Verification items for the finished model (mm, model axes). Face numbers are marked on the shaded views. A direction names the side the tool comes from. Give positions to 0.01 mm unless a question says otherwise; leave off trailing zeros. Loops run counter-clockwise (first coordinate to the right, second up) from the corner with the lowest first, then second, coordinate; pieces in that order, holes last. Notation, with made-up numbers: (80, 48) -> (133, 48) arc R31 cw to (133, 77) -> close; hole circle Ø4 at (79, 35.25). An arc over 180 degrees is marked (long way). Answer in a Markdown table with one row per item. Add a question column.
Q1. Gauge pin test, flat ends, axial feed: P1, Ø7.5, axis at x = 15.5, y = -41.5, coming from the -Z side; P2, Ø1.8, axis at x = 17, y = -42.5, coming from the +Z side; P3, Ø2, axis at x = -16.5, y = -1, coming from the -Z side; P4, Ø5, axis at y = -26.5, z = 3.5, coming from the +X side. Record the tip position at first contact, or that the pin passes through.
Q2. Material ranges on probe 1 along X at (y, z) = (-41.5, 4.85); probe 2 along Y at (x, z) = (-15.5, 1.35); probe 3 along Y at (x, z) = (0, 1.75), recorded low to high.
Q3. Section check D-D on y = -27.9. Enter the section's corners in (x, z).
Q4. Section check A-A on z = 20. Give the number of separate pieces and of enclosed holes in the cut face, and give its area (3 significant figures).
Q5. Release check for a two-part mould opening along Y. For the marked faces 1, 2, 3 and 4 record: pulls with the +Y half, pulls with the -Y half, needs draft (parallel to the pull), parting line crosses it, or undercut.
Q6. Section check B-B on z = 11.75. Enter the section's corners in (x, y) (3 decimals).
Q7. Set-up check for the marked faces 5, 6 and 7: record each of +Z, -Z, +X, -X, +Y, -Y from which the full face is reachable in a straight line by a thin tool's end or side.
```python
from build123d import *

# Parameters (mm, degrees)
SKETCH2_R           = 2.15
SKETCH2_R_2         = 1.804126588
SKETCH2_R_3         = 2.95
SKETCH2_W           = 9
SKETCH2_H           = 16
BOSS_EXTRUDE1_DEPTH = 3
SKETCH7_W           = 42.4
SKETCH7_H           = 70.4
SKETCH7_R           = 1.804126588
SKETCH7_R_2         = 2.95
BOSS_EXTRUDE4_DEPTH = 18
SKETCH3_W           = 42.4
SKETCH3_H           = 70.4
BOSS_EXTRUDE2_DEPTH = 5
CUT_EXTRUDE1_START  = -20
SKETCH4_R           = 2.95
CUT_EXTRUDE1_DEPTH  = 20
CUT_EXTRUDE2_REACH  = 71.96
SKETCH5_R           = 8
CUT_EXTRUDE3_START  = -11
SKETCH8_R           = 10.5
CUT_EXTRUDE3_DEPTH  = 2
CUT_EXTRUDE4_START  = -37.4
SKETCH8_2_R         = 10.5
CUT_EXTRUDE4_DEPTH  = 4.680146
CHAMFER1_SIZE       = 6
SKETCH6_R           = 3.95
BOSS_EXTRUDE3_DEPTH = 3
CHAMFER2_SIZE       = 0.25


with BuildPart() as part:
    # Sketch2 → Boss-Extrude1 (new body)
    # profile 1 of 4: a face of its own
    with BuildSketch(Plane.XY):
        with BuildLine():
            Line((21.2, -35.9), (12.2, -35.9))
            Line((12.2, -35.9), (12.2, -38.4))
            Line((12.2, -38.4), (12.2, -48.1))
            Line((12.2, -48.1), (-11.95, -48.1))
            Line((-11.95, -48.1), (-11.95, -40.891869727))
            Line((-11.95, -40.891869727), (-16.2, -37.241869727))
            Line((-16.2, -37.241869727), (-16.2, -19.819444087))
            Line((-16.2, -19.819444087), (-12.2, -15.659508007))
            Line((-12.2, -15.659508007), (-12.2, -14.172155799))
            ThreePointArc((-12.2, -14.172155799), (0, 18.7), (12.2, -14.172155799))
            Line((12.2, -14.172155799), (12.2, -17.4))
            Line((12.2, -17.4), (12.2, -19.9))
            Line((12.2, -19.9), (21.2, -19.9))
            Line((21.2, -19.9), (21.2, 21.2))
            Line((21.2, 21.2), (-13.2, 21.2))
            Line((-13.2, 21.2), (-21.2, 21.2))
            Line((-21.2, 21.2), (-21.2, -49.2))
            Line((-21.2, -49.2), (-9, -49.2))
            Line((-9, -49.2), (11.2, -49.2))
            Line((11.2, -49.2), (21.2, -49.2))
            Line((21.2, -49.2), (21.2, -35.9))
        make_face()
        with Locations((-15.5, -41.5)):
            Circle(SKETCH2_R, mode=Mode.SUBTRACT)
        with Locations((15.5, -41.5)):
            Circle(SKETCH2_R, mode=Mode.SUBTRACT)
        with Locations((-15.5, -15.5)):
            Circle(SKETCH2_R_2, mode=Mode.SUBTRACT)
        with Locations((-15.5, 15.5)):
            Circle(SKETCH2_R_3, mode=Mode.SUBTRACT)
        with Locations((15.5, -15.5)):
            Circle(SKETCH2_R_2, mode=Mode.SUBTRACT)
        with Locations((15.5, 15.5)):
            Circle(SKETCH2_R_3, mode=Mode.SUBTRACT)
    # profile 2 of 4: a face of its own
    with BuildSketch(Plane.XY):
        with Locations((16.7, -27.9)):
            Rectangle(SKETCH2_W, SKETCH2_H)
    # profile 3 of 4: a face of its own
    with BuildSketch(Plane.XY):
        with Locations((-15.5, -41.5)):
            Circle(SKETCH2_R)
        with Locations((-15.5, -41.5)):
            Circle(SKETCH2_R_2, mode=Mode.SUBTRACT)
    # profile 4 of 4: a face of its own
    with BuildSketch(Plane.XY):
        with Locations((15.5, -41.5)):
            Circle(SKETCH2_R)
        with Locations((15.5, -41.5)):
            Circle(SKETCH2_R_2, mode=Mode.SUBTRACT)
    extrude(amount=BOSS_EXTRUDE1_DEPTH)

    # Sketch7 → Boss-Extrude4 (add)
    with BuildSketch(Plane.XY.offset(3)):
        with Locations((0, -14)):
            Rectangle(SKETCH7_W, SKETCH7_H)
        with Locations((15.5, -41.5)):
            Circle(SKETCH7_R, mode=Mode.SUBTRACT)
        with Locations((-15.5, -41.5)):
            Circle(SKETCH7_R, mode=Mode.SUBTRACT)
        with Locations((-15.5, -15.5)):
            Circle(SKETCH7_R, mode=Mode.SUBTRACT)
        with Locations((15.5, -15.5)):
            Circle(SKETCH7_R, mode=Mode.SUBTRACT)
        with Locations((15.5, 15.5)):
            Circle(SKETCH7_R_2, mode=Mode.SUBTRACT)
        with Locations((-15.5, 15.5)):
            Circle(SKETCH7_R_2, mode=Mode.SUBTRACT)
        with BuildLine():
            Line((10.2, -46.1), (10.2, -13.223085873))
            ThreePointArc((10.2, -13.223085873), (0, 16.7), (-10.2, -13.223085873))
            Line((-10.2, -13.223085873), (-10.2, -16.465067137))
            Line((-10.2, -16.465067137), (-14.2, -20.625003217))
            Line((-14.2, -20.625003217), (-14.2, -36.323172457))
            Line((-14.2, -36.323172457), (-9.95, -39.973172457))
            Line((-9.95, -39.973172457), (-9.95, -46.1))
            Line((-9.95, -46.1), (10.2, -46.1))
        make_face(mode=Mode.SUBTRACT)
    extrude(amount=BOSS_EXTRUDE4_DEPTH)

    # Sketch3 → Boss-Extrude2 (add)
    with BuildSketch(Plane.XY.offset(21)):
        with Locations((0, -14)):
            Rectangle(SKETCH3_W, SKETCH3_H)
    extrude(amount=BOSS_EXTRUDE2_DEPTH)

    # Sketch4 → Cut-Extrude1 (cut)
    with BuildSketch(Plane.XY.offset(26).offset(CUT_EXTRUDE1_START)):
        with Locations((-15.5, -15.5)):
            Circle(SKETCH4_R)
        with Locations((15.5, -15.5)):
            Circle(SKETCH4_R)
        with Locations((-15.5, -41.5)):
            Circle(SKETCH4_R)
        with Locations((15.5, -41.5)):
            Circle(SKETCH4_R)
        with Locations((-15.5, 15.5)):
            Circle(SKETCH4_R)
        with Locations((15.5, 15.5)):
            Circle(SKETCH4_R)
    extrude(amount=CUT_EXTRUDE1_DEPTH, mode=Mode.SUBTRACT)

    # Sketch5 → Cut-Extrude2 (cut, up to next)
    with BuildSketch(Plane(origin=(21.2, 0, 0), x_dir=(0, 0, -1), z_dir=(1, 0, 0)), mode=Mode.PRIVATE) as cut_extrude2_sk1:
        with Locations((0, -27.9)):
            Circle(SKETCH5_R)
    cut_extrude2_tool1 = extrude(cut_extrude2_sk1.sketch, amount=-CUT_EXTRUDE2_REACH, mode=Mode.PRIVATE) & part.part
    add(cut_extrude2_tool1.solids().sort_by_distance((21.2, -27.9, 0))[0], mode=Mode.SUBTRACT)

    # Sketch8 → Cut-Extrude3 (cut)
    with BuildSketch(Plane(origin=(21.2, 0, 0), x_dir=(0, 0, -1), z_dir=(1, 0, 0)).offset(CUT_EXTRUDE3_START)):
        with Locations((0, -27.9)):
            Circle(SKETCH8_R)
    extrude(amount=CUT_EXTRUDE3_DEPTH, mode=Mode.SUBTRACT)

    # Sketch8<2> → Cut-Extrude4 (cut)
    with BuildSketch(Plane(origin=(21.2, 0, 0), x_dir=(0, 0, -1), z_dir=(1, 0, 0)).offset(CUT_EXTRUDE4_START)):
        with Locations((0, -27.9)):
            Circle(SKETCH8_2_R)
    extrude(amount=CUT_EXTRUDE4_DEPTH, mode=Mode.SUBTRACT)

    # Chamfer1
    chamfer1_edges = [part.edges().sort_by_distance(p)[0] for p in [
        (-21.2, 21.2, 13),
    ]]
    chamfer(chamfer1_edges, length=CHAMFER1_SIZE)

    # Sketch6 → Boss-Extrude3 (add)
    with BuildSketch(Plane(origin=(0, 0, 21), x_dir=(-1, 0, 0), z_dir=(0, 0, -1))):
        with Locations(Location((0, 0, 0), (0, 0, 180))):
            Circle(SKETCH6_R)
    extrude(amount=BOSS_EXTRUDE3_DEPTH)

    # Chamfer2
    chamfer2_edges = [part.edges().sort_by_distance(p)[0] for p in [
        (-3.95, 0, 18),
    ]]
    chamfer(chamfer2_edges, length=CHAMFER2_SIZE)


solid = part.part
```
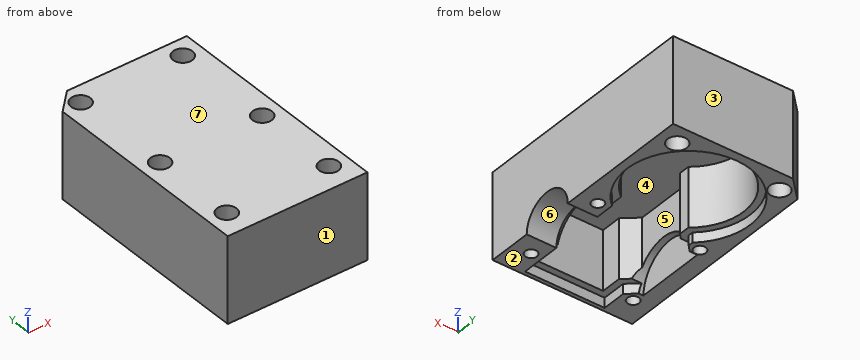
Taken from the geometry:
| question | item | result |
|---|---|---|
| 1 | P1 | stops at z = 0 |
| 1 | P2 | stops at z = 6 |
| 1 | P3 | stops at z = 3 |
| 1 | P4 | stops at x = -16.2 |
| 2 | probe 1 | x = -21.2 to -17.3, -13.7 to -9.95, 10.2 to 13.7, 17.3 to 21.2 |
| 2 | probe 2 | y = -49.2 to -43.3, -39.7 to -38.31, -17.49 to -17.3, -13.7 to -10.46, 10.46 to 12.55, 18.45 to 20.9 |
| 2 | probe 3 | y = -49.2 to -48.1, 18.7 to 21.2 |
| 3 | outline | (-21.2, 0) -> (-16.2, 0) -> (-16.2, 10.5) -> (-14.2, 10.5) -> (-14.2, 21) -> (10.2, 21) -> (10.2, 10.5) -> (12.2, 10.5) -> (12.2, 8) -> (21.2, 8) -> (21.2, 26) -> (-21.2, 26) -> close |
| 4 | separate pieces | 2 |
| 4 | enclosed holes | 7 |
| 4 | area | 1,280 mm² |
| 5 | face 1 | pulls with the -Y half |
| 5 | face 2 | needs draft |
| 5 | face 3 | pulls with the +Y half |
| 5 | face 4 | undercut |
| 6 | outline | (-21.2, -49.2) -> (21.2, -49.2) -> (21.2, 21.2) -> (-15.2, 21.2) -> (-21.2, 15.2) -> close; hole circle Ø5.9 at (-15.5, -41.5); hole circle Ø5.9 at (-15.5, -15.5); hole circle Ø5.9 at (-15.5, 15.5); hole (-14.2, -36.323) -> (-9.95, -39.973) -> (-9.95, -46.1) -> (10.2, -46.1) -> (10.2, -13.223) arc R16.7 ccw (long way) to (-10.2, -13.223) -> (-10.2, -16.465) -> (-14.2, -20.625) -> close; hole circle Ø5.9 at (15.5, -41.5); hole circle Ø5.9 at (15.5, -15.5); hole circle Ø5.9 at (15.5, 15.5) |
| 7 | face 5 | -Z |
| 7 | face 6 | -Z, +X |
| 7 | face 7 | +Z, +X, -X, +Y, -Y |
